from build123d import *

# Parameters (mm, degrees)
F0_R     = 1.881022
F0_R_2   = 1.942209
F1_DEPTH = 5


with BuildPart() as f1:
    # F0 (on Top) → F1 (new body)
    with BuildSketch(Plane.XY):
        with BuildLine():
            ThreePointArc((-10.141898, 9.43031), (-14.818735, 5.412834), (-10.570469, 0.944595))
            Line((-10.570469, 0.944595), (7.000959, 0.944595))
            ThreePointArc((7.000959, 0.944595), (9.553028, 2.109944), (10.343815, 4.801738))
            Line((10.343815, 4.801738), (10.343815, 19.801738))
            ThreePointArc((10.343815, 19.801738), (6.958101, 23.187452), (3.572387, 19.801738))
            add(Edge.make_bspline(
                [(3.572387, 9.43031), (3.572387, 12.887452), (3.572387, 16.344595), (3.572387, 19.801738)],
                knots=[0, 0, 0, 0, 10.371429, 10.371429, 10.371429, 10.371429], degree=3))
            add(Edge.make_bspline(
                [(-10.141898, 9.43031), (-5.570469, 9.43031), (-0.999041, 9.43031), (3.572387, 9.43031)],
                knots=[0, 0, 0, 0, 13.714285, 13.714285, 13.714285, 13.714285], degree=3))
        make_face()
        with Locations((-10.570469, 5.198275)):
            Circle(F0_R, mode=Mode.SUBTRACT)
        with Locations((6.958101, 19.801738)):
            Circle(F0_R_2, mode=Mode.SUBTRACT)
    extrude(amount=F1_DEPTH)


solid = f1.part
CAD build for the part. Positions are in the model's coordinates, mm. A direction names the side the tool comes from. Coordinates: 2 decimals unless noted, no trailing zeros. Order: outer loops, then holes, each group sorted by start corner. A loop starts at its lowest first (then second) coordinate and runs counter-clockwise, first axis right, second up.
Item 1: Drill centre lines: L1, parallel to Y at x = -0.5, z = 0.9; L2, parallel to X at y = 15, z = 2.75; L3, parallel to X at y = 6, z = 0.65. Where is each one in solid material? Low to high.
Check sheet entries:
L1: y = 0.94 to 9.43
L2: x = 3.57 to 10.34
L3: x = -14.75 to -12.27, -8.87 to 10.34
Item 2: Band-saw the part on A-A on y = 4.25. List the corners of the cut face in (x, z).
Check sheet entries:
outline: (-14.72, 0) - (-12.19, 0) - (-12.19, 5) - (-14.72, 5) - close; (-8.95, 0) - (10.38, 0) - (10.38, 5) - (-8.95, 5) - close
Item 3: Two-plate mould, pull along X, no slides. Class faces 3 (the face through (0, 7, 5)), 4 (the face through (5.417, 18.62, 2.465)), 5 (the face through (9.526, 2.079, 2.465)): +X half, -X half, draft (parallel to the pull), parting line (faces both ways), or undercut.
Check sheet entries:
face 3: draft
face 4: undercut
face 5: +X half
Item 4: Pin check, flat tip, straight feed: pin 1 Ø2 at (y, z) = (17, 0.5) entering from -X. Stop position of the tip, or through.
Check sheet entries:
pin 1: stops at x = 3.57
Item 5: 3-axis set-ups, long thin cutter, end or side, ignore diameter. For faces 1 (the face through (10.344, 12, 2)), 2 (the face through (0, 7, 0)): which of +Z, -Z, +X, -X, +Y, -Y reach the whole face in a straight line?
Check sheet entries:
face 1: +Z, -Z, +X, +Y
face 2: -Z, +X, -X, +Y, -Y
Item 6: Band-saw the part on C-C on z = 2.1. Give the number of separate pieces and of enclosed holes in the cut face, plus the area to 3 significant figures.
Check sheet entries:
separate pieces: 1
enclosed holes: 2
area: 269 mm2
Item 7: Band-saw the part on B-B on x = 6.25. List the corners of the cut face in (y, z).
Check sheet entries:
outline: (0.94, 0) - (17.99, 0) - (17.99, 5) - (0.94, 5) - close; (21.61, 0) - (23.11, 0) - (23.11, 5) - (21.61, 5) - close
